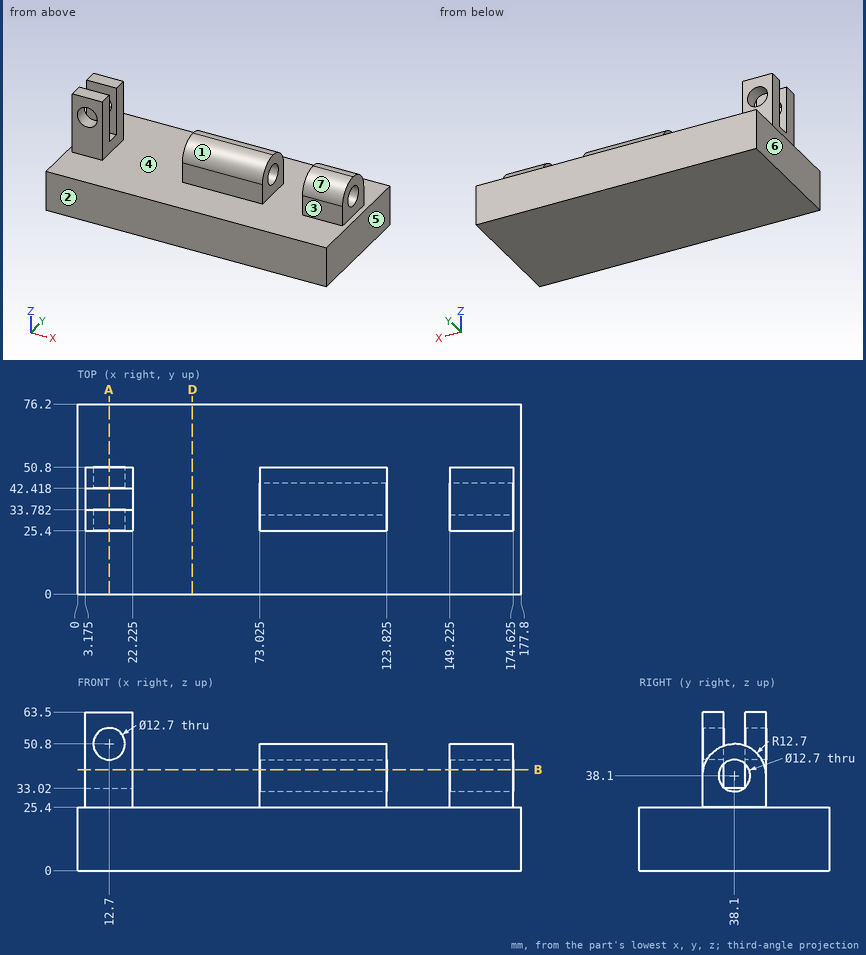
For this review, use the dimensioned drawing (mm, ordinates from the lowest corner) and the shaded views. A direction names the side the tool comes from. Coordinates: 2 decimals unless noted, no trailing zeros. Write each loop counter-clockwise with the first axis right and the second up, starting at its lowest first coordinate (ties: lowest second). Pieces come first, ordered by that corner, then holes. Notation, with made-up numbers: (-20, -15) -> (-5, -15) arc R17 ccw to (-5, 17) -> close; hole circle Ø11 at (45.25, -14.75). An arc over 180 degrees is marked (long way). Put each result on its own line as item: value.
Q1. Take a section at B-B, the plane z = 40.5. State the section outline as (x, y) points (3 decimals).
From the geometry:
outline: (3.175, 25.4) -> (22.225, 25.4) -> (22.225, 33.782) -> (3.175, 33.782) -> close; (3.175, 42.418) -> (22.225, 42.418) -> (22.225, 50.8) -> (3.175, 50.8) -> close; (73.025, 25.629) -> (123.825, 25.629) -> (123.825, 32.221) -> (73.025, 32.221) -> close; (73.025, 43.979) -> (123.825, 43.979) -> (123.825, 50.571) -> (73.025, 50.571) -> close; (149.225, 25.629) -> (174.625, 25.629) -> (174.625, 32.221) -> (149.225, 32.221) -> close; (149.225, 43.979) -> (174.625, 43.979) -> (174.625, 50.571) -> (149.225, 50.571) -> close
Q2. Tool access review of the marked faces 1, 2 and 3: name each direction out of +Z, -Z, +X, -X, +Y, -Y from which nothing blocks a thin tool from reaching the whole face with its end or side.
From the geometry:
face 1: +Z, +X, -Y
face 2: +Z, -Z, +X, -X, -Y
face 3: +Z, +X, -X, -Y
Q3. Take a section at A-A, the plane x = 12.7. State the section outline as (y, z) points.
From the geometry:
outline: (0, 0) -> (76.2, 0) -> (76.2, 25.4) -> (50.8, 25.4) -> (50.8, 44.45) -> (42.42, 44.45) -> (42.42, 33.02) -> (33.78, 33.02) -> (33.78, 44.45) -> (25.4, 44.45) -> (25.4, 25.4) -> (0, 25.4) -> close; (25.4, 57.15) -> (33.78, 57.15) -> (33.78, 63.5) -> (25.4, 63.5) -> close; (42.42, 57.15) -> (50.8, 57.15) -> (50.8, 63.5) -> (42.42, 63.5) -> close
Q4. Take a section at D-D, the plane x = 46. State the section outline as (y, z) points.
From the geometry:
outline: (0, 0) -> (76.2, 0) -> (76.2, 25.4) -> (0, 25.4) -> close
Q5. Wall thickness on L1, parallel to Z at x = 12.7, y = 27.75; L2, parallel to Z at x = 164, y = 38; L3, parallel to Z at x = 29, y = 47: over which ranges is each line inside the solid? List them lowest first.
From the geometry:
L1: z = 0 to 44.45, 57.15 to 63.5
L2: z = 0 to 31.75, 44.45 to 50.8
L3: z = 0 to 25.4
Q6. Clearance check with flat-ended pins moving along their axes: pin 1 Ø6.5 at (x, z) = (103, 32.5) entering from -Y; pin 2 Ø7.5 at (y, z) = (33, 47.5) entering from +X (3 decimals); pin 3 Ø15 at (x, z) = (8.5, 39.5) entering from +Y. State where each tip first meets the part, or that it passes through.
From the geometry:
pin 1: stops at y = 25.4
pin 2: stops at x = 174.625
pin 3: stops at y = 50.8
Q7. The part is to be moulded in two halves that separate along X. For the marked faces 4, 5, 6 and 7, say which applies: +X half, -X half, draft (parallel to the pull), parting line (faces both ways), or undercut.
From the geometry:
face 4: undercut
face 5: +X half
face 6: -X half
face 7: draft
